Autodesk Inventor part; units mm, degrees
ref_plane "YZ Plane" through (0, 0, 0) normal (1, 0, 0) x (0, 1, 0)
ref_plane "XZ Plane" through (0, 0, 0) normal (0, 1, 0) x (-1, 0, 0)
ref_plane "XY Plane" through (0, 0, 0) normal (0, 0, 1) x (1, 0, 0)
sketch "Sketch1" plane through (0, 0, 0) normal (0, 0, 1) x (1, 0, 0)
  line L0 (-18.5, -6) -> (18.5, -6)
  line L1 (18.5, -6) -> (18.5, 6)
  line L2 (18.5, 6) -> (-18.5, 6)
  line L3 (-18.5, 6) -> (-18.5, -6)
  line L4 (-18.5, -6) -> (18.5, 6) construction
  line L5 (18.5, -6) -> (-18.5, 6) construction
  point P0 (0, 0)
  dimension "d0" = 37
  dimension "d1" = 12
extrude "Extrusion1" add sketch "Sketch1" along normal mid plane 5
sketch "Sketch2" plane through (-18.5, 6, 2.5) normal (0, 1, 0) x (1, 0, 0)
  line L0 (3.2, 5.874) -> (9.2, 5.874)
  line L1 (9.2, 5.874) -> (9.2, 4.874)
  line L2 (9.2, 4.874) -> (3.2, 4.874)
  line L3 (3.2, 4.874) -> (3.2, 5.874)
  line L4 (3.2, 5.874) -> (9.2, 4.874) construction
  line L5 (9.2, 5.874) -> (3.2, 4.874) construction
  line L6 (37, 5) -> (37, 0)
  line L7 (9.074, 5.748) -> (3.326, 5.748)
  line L8 (3.326, 5.748) -> (3.326, 5)
  line L9 (3.326, 5) -> (9.074, 5)
  line L10 (9.074, 5) -> (9.074, 5.748)
  line L11 (0, 5) -> (37, 5)
  point P0 (18.5, 2.5)
  point P1 (6.2, 5.374)
  dimension "d4" = 27.8
  dimension "d5" = 1
  dimension "d6" = 6
  dimension "d7" = 0.126
extrude "Extrusion2" add sketch "Sketch2" against normal up to surface (12 mm away) contours L8 L7 L10 L9
sketch "Sketch3" plane through (0, 0, 2.5) normal (0, 0, 1) x (1, 0, 0)
  line L0 (-18.5, -6) -> (18.5, -6)
  line L1 (-9.426, -6) -> (-15.174, -6)
  line L2 (-15.174, 6) -> (-15.174, -6)
  line L3 (-9.426, 6) -> (-15.174, 6)
  line L4 (-9.426, 6) -> (-9.426, -6)
  point P0 (0, 0)
  point P1 (-12.3, 0)
  point P2 (-12.3, 6)
  point P3 (-9.426, 0)
hole "Hole1" at (-12.3, 0, 2.5) direction (0, 0, -1) diameter 5.5 depth 14.2
fillet "Fillet1" radius 4 4 edges at (-18.5, 6, 0) (-18.5, -6, 0) (18.5, -6, 0) (18.5, 6, 0)
fillet "Fillet2" radius 1 8 edges at (-17.3284, 4.8284, 2.5) (-18.5, 0, 2.5) (-17.3284, -4.8284, 2.5) (0, -6, 2.5) (17.3284, -4.8284, 2.5) (18.5, 0, 2.5) (17.3284, 4.8284, 2.5) (0, 6, 2.5)
sketch "Sketch4" plane through (0, 0, -2.5) normal (0, 0, -1) x (-1, 0, 0)
  line L0 (-18.5, 2) -> (-18.5, -2)
  point P0 (0, 0)
  point P1 (-13.4, 0)
  point P2 (-3.9, 0)
  dimension "d19" = 5.1
  dimension "d20" = 14.6
hole "Hole2" at (13.4, 0, -2.5) at (3.9, 0, -2.5) direction (0, 0, 1) diameter 2.013 depth 7.6
properties part number "Frame_Z_Endstop_Mount_LM3048" material "ABS Plastic"
The listing builds one solid part. Answer for the finished solid, in the listing's coordinates (mm). A direction names the side the tool comes from. Round coordinates to 2 decimals unless told otherwise and drop trailing zeros. Loops run counter-clockwise (first coordinate to the right, second up) from the corner with the lowest first, then second, coordinate; pieces in that order, holes last.
1) Given P1, Ø1.2, axis at x = 13.4, y = 0, coming from the +Z side (1 decimal); P2, Ø2.5, axis at x = 3.9, y = 0, coming from the -Z side; P3, Ø0.6, axis at y = 2.5, z = -3, coming from the +X side; P4, Ø0.8, axis at y = -0.5, z = -3, coming from the -X side, each flat-ended and moving along its own axis, determine where each tip first touches the part or whether it passes through.
Outcome:
P1: passes through
P2: stops at z = -2.5
P3: stops at x = -9.43
P4: stops at x = -15.17
2) A cutting plane is placed at D-D on y = 1.5. Determine the outline of the cut face in (x, z), plus the area to 3 significant figures.
Outcome:
outline: (-18.5, -2.5) - (-15.17, -2.5) - (-15.17, -3.25) - (-14.6, -3.25) - (-14.6, 2.5) - (-17.5, 2.5) arc R1 ccw to (-18.5, 1.5) - close; (-10, -3.25) - (-9.43, -3.25) - (-9.43, -2.5) - (18.5, -2.5) - (18.5, 1.5) arc R1 ccw to (17.5, 2.5) - (-10, 2.5) - close
area: 162 mm2
3) For a pull along X with two mould halves and no side action, classify faces 1 (the face through (2.9, -0.1, 0)), 2 (the face through (-9.615, 0.596, -0.414)), 3 (the face through (-18.5, 0, -1)), 4 (the face through (17.297, -4.859, -0.472)) as released by +X, released by -X, zero draft, split by the parting line, or undercut.
Outcome:
face 1: undercut
face 2: undercut
face 3: released by -X
face 4: released by +X
4) A cutting plane is placed at C-C on z = -0.8. Determine the outline of the cut face in (x, y), plus the area to 3 significant figures.
Outcome:
outline: (-18.5, -2) arc R4 ccw to (-14.5, -6) - (14.5, -6) arc R4 ccw to (18.5, -2) - (18.5, 2) arc R4 ccw to (14.5, 6) - (-14.5, 6) arc R4 ccw to (-18.5, 2) - close; hole circle Ø5.5 at (-12.3, 0); hole circle Ø2.01 at (3.9, 0); hole circle Ø2.01 at (13.4, 0)
area: 400 mm2
5) For faces 5 (the face through (4.3, -1.2, -2.5)), 6 (the face through (-12, 3, -3.248)), 7 (the face through (-17, 0, -2.5)), determine the directions among +Z, -Z, +X, -X, +Y, -Y from which every point of the face is accessible in a straight line to the end or side of a thin tool.
Outcome:
face 5: -Z, +X, +Y, -Y
face 6: -Z, +X, -X, +Y, -Y
face 7: -Z, -X, +Y, -Y
6) Consider line 1 (X direction, y = 0, z = 0.5); line 2 (Y direction, x = -12.3, z = -0.7); line 3 (Y direction, x = 13.4, z = -0.65). Determine where each line is inside the solid, lowest interval first.
Outcome:
line 1: x = -18.5 to -15.05, -9.55 to 2.89, 4.91 to 12.39, 14.41 to 18.5
line 2: y = -6 to -2.75, 2.75 to 6
line 3: y = -6 to -1.01, 1.01 to 6
7) A cutting plane is placed at B-B on x = 3.9. Determine the outline of the cut face in (y, z), plus the area to 3 significant figures.
Outcome:
outline: (-6, -2.5) - (-1.01, -2.5) - (-1.01, 2.5) - (-5, 2.5) arc R1 ccw to (-6, 1.5) - close; (1.01, -2.5) - (6, -2.5) - (6, 1.5) arc R1 ccw to (5, 2.5) - (1.01, 2.5) - close
area: 49.5 mm2
8) A cutting plane is placed at A-A on y = 0. Determine the outline of the cut face in (x, z), plus the area to 3 significant figures.
Outcome:
outline: (-18.5, -2.5) - (-15.17, -2.5) - (-15.17, -3.25) - (-15.05, -3.25) - (-15.05, 2.5) - (-17.5, 2.5) arc R1 ccw to (-18.5, 1.5) - close; (-9.55, -3.25) - (-9.43, -3.25) - (-9.43, -2.5) - (2.89, -2.5) - (2.89, 2.5) - (-9.55, 2.5) - close; (4.91, -2.5) - (12.39, -2.5) - (12.39, 2.5) - (4.91, 2.5) - close; (14.41, -2.5) - (18.5, -2.5) - (18.5, 1.5) arc R1 ccw to (17.5, 2.5) - (14.41, 2.5) - close
area: 137 mm2
